from build123d import *

# Parameters (mm, degrees)
F0_W     = 88.9
F0_H     = 73.025
F1_DEPTH = 25.4
F2_T     = -2.54
F3_W     = 12.7
F3_H     = 9.525
F3_R     = 3.96875
F4_DEPTH = 2.54


with BuildPart() as f1:
    # F0 (on Top) → F1 (new body)
    with BuildSketch(Plane.XY):
        with Locations((44.45, 36.5125)):
            Rectangle(F0_W, F0_H)
    extrude(amount=F1_DEPTH)

    # F2
    f2_openings = [f1.faces().sort_by_distance(p)[0] for p in [
        (44.45, 36.5125, 25.4),
    ]]
    offset(amount=F2_T, openings=f2_openings)

    # F3 (on face) → F4 (cut)
    with BuildSketch(Plane.YZ.offset(88.9)):
        with Locations((15.723732, 15.242798)):
            Rectangle(F3_W, F3_H)
        with Locations((33.899404, 15.242798)):
            Circle(F3_R)
    extrude(amount=-F4_DEPTH, mode=Mode.SUBTRACT)


solid = f1.part
Design review of the part built by this model. Coordinates are the model's own, in mm. A direction names the side the tool comes from. Coordinates: 2 decimals unless noted, no trailing zeros. Loops run counter-clockwise (first coordinate to the right, second up) from the corner with the lowest first, then second, coordinate; pieces in that order, holes last. Notation, with made-up numbers: (-24.75, 35) - (22.25, 35) arc R13 ccw to (22.25, 46) - close; hole circle Ø6 at (80.5, 89). An arc over 180 degrees is marked (long way). Use CSV: the item, a comma, the result in double quotes. Start each with the question number.
1. Clearance check with a flat-ended pin moving along its axis: pin 1 (2 mm diameter, centred on x = 34, y = 41.5, fed in from +Z). State where the tip first meets the part, or that it passes through.
2. Add section A-A on z = 6.25. Give the boundary of the cut face in (x, y) (3 decimals), plus the area to 3 significant figures.
3. Add section D-D on z = 12.25. Give the boundary of the cut face in (x, y) (3 decimals), plus the area to 3 significant figures.
4. Add section C-C on x = 16.5. Give the boundary of the cut face in (y, z) (3 decimals).
5. Mouldability with a two-part tool opening along Y and no side actions: class faces 4 (the flat face through (44, 37, 2.54)), 5 (the flat face through (44, 73.025, 13)), 6 (the flat face through (44, 37, 0)), 7 (the flat face through (44, 0, 13)) as released by +Y, released by -Y, zero draft, split by the parting line, or undercut.
6. Add section B-B on y = 10.5. Give the boundary of the cut face in (x, z).
7. For faces 1 (the flat face through (86.36, 36, 11)), 2 (the flat face through (88, 16, 10.48)), 3 (the flat face through (88.9, 36, 10)), list the 3-axis set-ups (+Z, -Z, +X, -X, +Y, -Y) from which the entire face can be reached by the end or side of a thin tool; tool diameter is ignored.
8. To check wall thickness, follow probe 1 along Y at (x, z) = (10, 18.5) (3 decimals); probe 2 along X at (y, z) = (66, 10.75); probe 3 along Z at (x, y) = (43, 29.5). State the ranges of each line that lie inside material, in increasing order.
Resolved:
1,pin 1,"z = 2.54"
2,outline,"(0, 0) - (88.9, 0) - (88.9, 73.025) - (0, 73.025) - close; hole (2.54, 2.54) - (86.36, 2.54) - (86.36, 70.485) - (2.54, 70.485) - close"
2,area,"797 mm2"
3,outline,"(0, 0) - (88.9, 0) - (88.9, 9.374) - (86.36, 9.374) - (86.36, 2.54) - (2.54, 2.54) - (2.54, 70.485) - (86.36, 70.485) - (86.36, 36.506) - (88.9, 36.506) - (88.9, 73.025) - (0, 73.025) - close; (86.36, 22.074) - (88.9, 22.074) - (88.9, 31.293) - (86.36, 31.293) - close"
3,area,"751 mm2"
4,outline,"(0, 0) - (73.025, 0) - (73.025, 25.4) - (70.485, 25.4) - (70.485, 2.54) - (2.54, 2.54) - (2.54, 25.4) - (0, 25.4) - close"
5,face 4,"undercut"
5,face 5,"released by +Y"
5,face 6,"zero draft"
5,face 7,"released by -Y"
6,outline,"(0, 0) - (88.9, 0) - (88.9, 10.48) - (86.36, 10.48) - (86.36, 2.54) - (2.54, 2.54) - (2.54, 25.4) - (0, 25.4) - close; (86.36, 20.01) - (88.9, 20.01) - (88.9, 25.4) - (86.36, 25.4) - close"
7,face 1,"+Z"
7,face 2,"+X"
7,face 3,"+Z, -Z, +X, +Y, -Y"
8,probe 1,"0 to 2.54, 70.485 to 73.025"
8,probe 2,"0 to 2.54, 86.36 to 88.9"
8,probe 3,"0 to 2.54"
